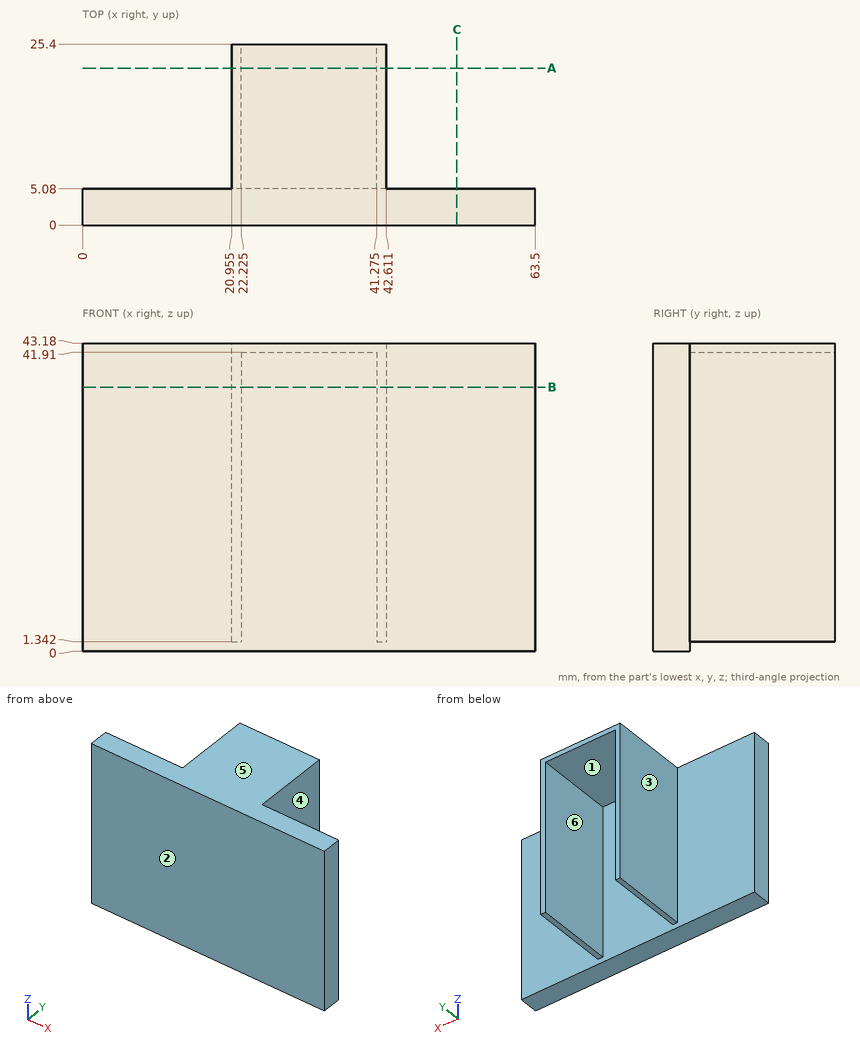
Study the drawing (mm; zero at the part's minimum x, y, z) and answer. A direction names the side the tool comes from. Coordinates: 2 decimals unless noted, no trailing zeros. Write each loop counter-clockwise with the first axis right and the second up, starting at its lowest first coordinate (ties: lowest second). Pieces come first, ordered by that corner, then holes.
Q1. A cutting plane is placed at C-C, the plane x = 52.5. Give the vertices of the cut face in (y, z), then the cut area to 3 significant figures.
Q2. Which of the six approach directions +Z, -Z, +X, -X, +Y, -Y give full straight-line access (tool end or side, diameter ignored) to the marked faces 1 and 2?
Q3. A cutting plane is placed at B-B, the plane z = 37. Give the vertices of the cut face in (x, y) (3 decimals).
Q4. Determine the mould class of the marked faces 3, 4, 5 and 6 for opening direction X: released by +X, released by -X, zero draft, split by the parting line, or undercut.
Q5. Find the intervals of material crossed by line 1 (X direction, y = 15, z = 34) (3 decimals); line 2 (Z direction, x = 25, y = 16); line 3 (Y direction, x = 46, z = 15), in increasing order.
Q6. Each of these flat-tipped pins is pushed along its axis until it touches: pin 1 Ø1 at (x, z) = (27, 6) entering from -Y; pin 2 Ø1.1 at (x, y) = (41.5, 17.5) entering from -Z; pin 3 Ø6 at (y, z) = (15, 15.5) entering from +X. Where does it stop, or does it pass through?
Q7. A cutting plane is placed at A-A, the plane y = 22. Give the vertices of the cut face in (x, z) (3 decimals), then the cut area to 3 significant figures.
Findings below:
1. outline: (0, 0) - (5.08, 0) - (5.08, 43.18) - (0, 43.18) - close
1. area: 219 mm2
2. face 1: -Z, +Y
2. face 2: +Z, -Z, +X, -X, -Y
3. outline: (0, 0) - (63.5, 0) - (63.5, 5.08) - (42.611, 5.08) - (42.611, 25.4) - (41.275, 25.4) - (41.275, 5.08) - (22.225, 5.08) - (22.225, 25.4) - (20.955, 25.4) - (20.955, 5.08) - (0, 5.08) - close
4. face 3: released by -X
4. face 4: released by +X
4. face 5: zero draft
4. face 6: undercut
5. line 1: x = 20.955 to 22.225, 41.275 to 42.611
5. line 2: z = 41.91 to 43.18
5. line 3: y = 0 to 5.08
6. pin 1: stops at y = 0
6. pin 2: stops at z = 1.34
6. pin 3: stops at x = 42.61
7. outline: (20.955, 1.342) - (22.225, 1.342) - (22.225, 41.91) - (41.275, 41.91) - (41.275, 1.342) - (42.611, 1.342) - (42.611, 43.18) - (20.955, 43.18) - close
7. area: 133 mm2
